```python
from build123d import *

# Parameters (mm, degrees)
F0_W     = 4.445
F0_H     = 69.088
F1_DEPTH = 42.545
F2_W     = 43.18
F2_H     = 69.088
F3_DEPTH = 4.445
F4_W     = 13.335
F4_H     = 4.445
F5_DEPTH = 13.335
F7_DEPTH = 4.445


with BuildPart() as f1:
    # F0 (on Front) → F1 (new body)
    with BuildSketch(Plane.XZ):
        with Locations((2.2225, 34.544)):
            Rectangle(F0_W, F0_H)
    extrude(amount=F1_DEPTH)

    # F2 (on Front) → F3 (join)
    with BuildSketch(Plane.XZ):
        with Locations((26.035, 34.544)):
            Rectangle(F2_W, F2_H)
    extrude(amount=F3_DEPTH)

    # F4 (on Front) → F5 (join)
    with BuildSketch(Plane.XZ):
        with Locations((6.6675, -2.2225)):
            Rectangle(F4_W, F4_H)
    extrude(amount=F5_DEPTH)

    # F6 (on face) → F7 (join)
    with BuildSketch(Plane.XY.offset(69.088)):
        with BuildLine():
            Line((47.625, 0), (0, 0))
            Line((0, 0), (0, -42.545))
            Line((0, -42.545), (10.795, -42.545))
            Line((10.795, -42.545), (10.795, -20.955))
            ThreePointArc((10.795, -20.955), (20.955, -10.795), (31.115, -20.955))
            Line((31.115, -20.955), (31.115, -42.545))
            Line((31.115, -42.545), (47.625, -42.545))
            Line((47.625, -42.545), (47.625, 0))
        make_face()
    extrude(amount=F7_DEPTH)


solid = f1.part
```
Part model, mm, in its own coordinate system. A direction names the side the tool comes from. Give positions to 0.01 mm unless a question says otherwise; leave off trailing zeros. Order: outer loops, then holes, each group sorted by start corner. A loop starts at its lowest first (then second) coordinate and runs counter-clockwise, first axis right, second up. Notation, with made-up numbers: (-24.75, -16.5) - (9.25, -16.5) arc R14 cw to (9.25, 8.5) - close; hole circle Ø8 at (-21.75, 48.25). An arc over 180 degrees is marked (long way). Use one line per item in the form item = value.
Item 1: Slice it at A-A on y = -37.5. Give the cut face in (x, z) (3 decimals), and give its area (3 significant figures).
Solution:
outline = (0, 0) - (4.445, 0) - (4.445, 69.088) - (10.795, 69.088) - (10.795, 73.533) - (0, 73.533) - close; (31.115, 69.088) - (47.625, 69.088) - (47.625, 73.533) - (31.115, 73.533) - close
area = 428 mm2
Item 2: Slice it at B-B on y = -7. Give the cut face in (x, z) (3 decimals), and give its area (3 significant figures).
Solution:
outline = (0, -4.445) - (13.335, -4.445) - (13.335, 0) - (4.445, 0) - (4.445, 69.088) - (47.625, 69.088) - (47.625, 73.533) - (0, 73.533) - close
area = 578 mm2
Item 3: Slice it at D-D on x = 7.5. Give the cut face in (y, z) (3 decimals).
Solution:
outline = (-42.545, 69.088) - (-4.445, 69.088) - (-4.445, 0) - (-13.335, 0) - (-13.335, -4.445) - (0, -4.445) - (0, 73.533) - (-42.545, 73.533) - close
Item 4: Probe probe 1 along Z at (x, y) = (12.5, -12) (3 decimals); probe 2 along Y at (x, z) = (10.5, 10.5) (3 decimals); probe 3 along Z at (x, y) = (7, -14.5). List the from-to ranges inside material, lowest first. Write a range as from..to.
Solution:
probe_1 = -4.445..0, 69.088..73.533
probe_2 = -4.445..0
probe_3 = 69.09..73.53
Item 5: Which spindle directions (+Z, -Z, +X, -X, +Y, -Y) get a long thin tool onto all of the face, cutting with end or side? Do faces 5 (the face through (31.115, -32, 71)), 6 (the face through (39, -42.545, 71)), 7 (the face through (9, -9, 0)), 8 (the face through (2, -28, 0)), 9 (the face through (30, -2, 0)). Say none if no direction does.
Solution:
face_5 = +Z, -Z, -Y
face_6 = +Z, -Z, +X, -X, -Y
face_7 = +X, -Y
face_8 = -Z, +X, -X, -Y
face_9 = -Z, +X, +Y, -Y
Item 6: Pin check, flat tips, straight feed: pin 1 Ø13 at (x, z) = (23, 19) entering from -Y (3 decimals); pin 2 Ø12 at (x, y) = (5.5, -29) entering from -Z; pin 3 Ø3 at (y, z) = (-22, 55) entering from +X (3 decimals); pin 4 Ø12 at (x, y) = (22, -19) entering from +Z. Stop position of each tip, or through.
Solution:
pin_1 = -4.445
pin_2 = 0
pin_3 = 4.445
pin_4 = through
Item 7: Slice it at C-C on z = 25.5. Give the cut face in (x, y) (3 decimals).
Solution:
outline = (0, -42.545) - (4.445, -42.545) - (4.445, -4.445) - (47.625, -4.445) - (47.625, 0) - (0, 0) - close
Item 8: Two-plate mould, pull along Z, no slides. Class faces 1 (the face through (13.335, -7, -2)), 2 (the face through (29, -12, 73.533)), 3 (the face through (26, -4.445, 35)), 4 (the face through (4.445, -23, 34)): released by +Z, released by -Z, zero draft, split by the parting line, or undercut.
Solution:
face_1 = zero draft
face_2 = released by +Z
face_3 = undercut
face_4 = undercut
